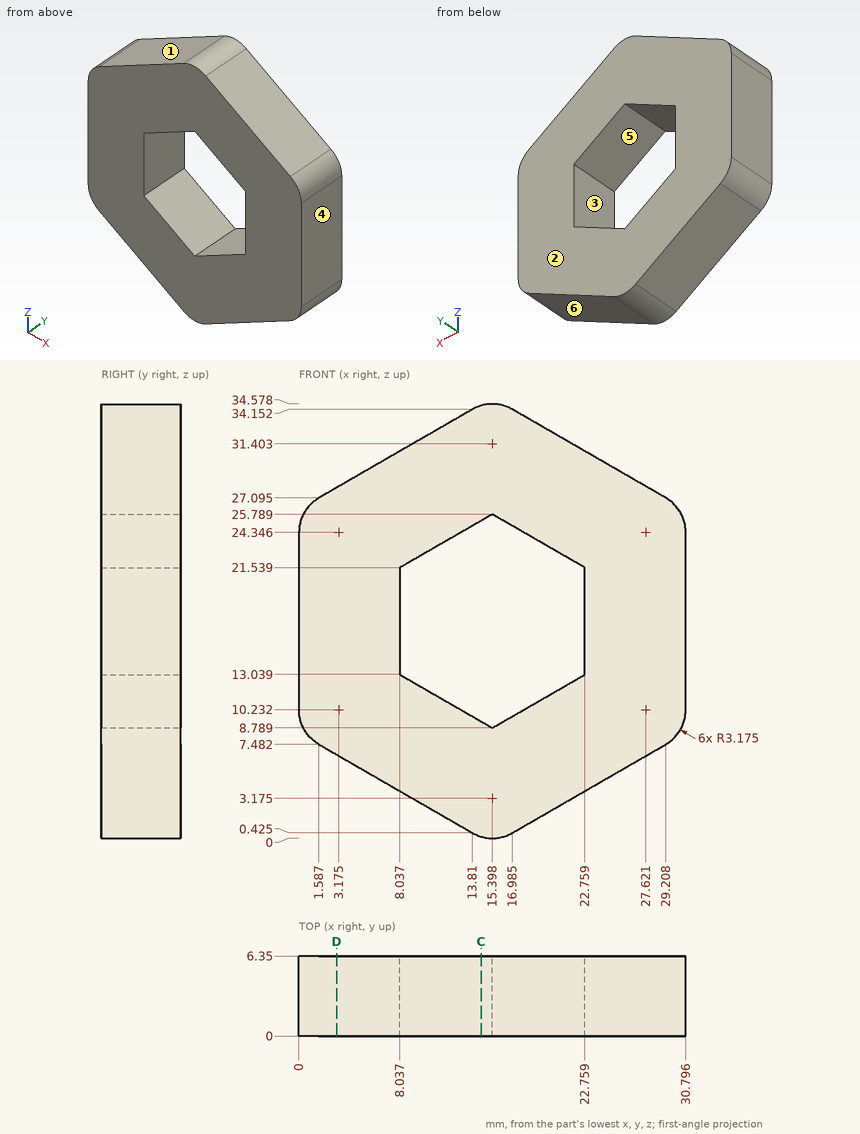
Verification items for this drawing (mm, ordinates from the low corner). A direction names the side the tool comes from. Coordinates: 2 decimals unless noted, no trailing zeros. Loops run counter-clockwise (first coordinate to the right, second up) from the corner with the lowest first, then second, coordinate; pieces in that order, holes last.
Item 1: Thickness scan on line 1 (X direction, y = 1.25, z = 19.5) (1 decimal); line 2 (X direction, y = 4.25, z = 22.5) (1 decimal); line 3 (Z direction, x = 10, y = 2) (1 decimal). Record the ranges inside material, lowest first.
Item 2: Release check for a two-part mould opening along X. For the marked faces 1, 2, 3 and 4 record: released by +X, released by -X, zero draft, split by the parting line, or undercut.
Item 3: Access from +Z, -Z, +X, -X, +Y, -Y to the whole of each face (thin tool, end or side, straight path). Record for the marked faces 5 and 6.
Item 4: Go/stop test with a flat-tipped pin: pin 1 Ø1.5 at (x, y) = (7, 4) entering from +Z. Record where the tip stops, or that it passes through.
Item 5: Sectioned sample at D-D, the plane x = 3. Record the boundary of the cut face in (y, z), then the cut area to 3 significant figures.
Item 6: Sectioned sample at C-C, the plane x = 14.5. Record the boundary of the cut face in (y, z).
Check result:
1. line 1: x = 0 to 8, 22.8 to 30.8
1. line 2: x = 0 to 9.7, 21.1 to 30.8
1. line 3: z = 2.6 to 11.9, 22.7 to 32
2. face 1: released by -X
2. face 2: zero draft
2. face 3: undercut
2. face 4: released by +X
3. face 5: +Y, -Y
3. face 6: -Z, +X, +Y, -Y
4. pin 1: stops at z = 30.65
5. outline: (0, 6.67) - (6.35, 6.67) - (6.35, 27.91) - (0, 27.91) - close
5. area: 135 mm2
6. outline: (0, 0.13) - (6.35, 0.13) - (6.35, 9.31) - (0, 9.31) - close; (0, 25.27) - (6.35, 25.27) - (6.35, 34.45) - (0, 34.45) - close
